from build123d import *

# Parameters (mm, degrees)
CROQUIS1_R              = 6
CROQUIS1_R_2            = 3
SALIENTE_EXTRUIR1_DEPTH = 2.5
CROQUIS3_W              = 4
CROQUIS3_H              = 4
CROQUIS3_R              = 0.75
SALIENTE_EXTRUIR2_DEPTH = 2.5
CORTAR_EXTRUIR1_DEPTH   = 5
MATRIZC1_COUNT          = 3


with BuildPart() as part:
    # Croquis1 → Saliente-Extruir1 (new, symmetric)
    with BuildSketch(Plane.XY):
        Circle(CROQUIS1_R)
        Circle(CROQUIS1_R_2, mode=Mode.SUBTRACT)
    extrude(amount=SALIENTE_EXTRUIR1_DEPTH, both=True)

    # Croquis3 → Saliente-Extruir2 (add, symmetric)
    with BuildSketch(Plane(origin=(0, 0, 0), x_dir=(0, 0, -1), z_dir=(1, 0, 0))):
        with Locations((0, 7)):
            Rectangle(CROQUIS3_W, CROQUIS3_H)
        with Locations((0, 7.5)):
            Circle(CROQUIS3_R, mode=Mode.SUBTRACT)
    saliente_extruir2 = extrude(amount=SALIENTE_EXTRUIR2_DEPTH, both=True)

    # Croquis4 → Cortar-Extruir1 (cut)
    with BuildSketch(Plane.XY.offset(2)):
        with BuildLine():
            Line((-1.25, 9), (1.25, 9))
            Line((1.25, 9), (1.25, 7.5))
            ThreePointArc((1.25, 7.5), (0.957106781, 6.792893219), (0.25, 6.5))
            Line((0.25, 6.5), (-0.25, 6.5))
            ThreePointArc((-0.25, 6.5), (-0.957106781, 6.792893219), (-1.25, 7.5))
            Line((-1.25, 7.5), (-1.25, 9))
        make_face()
    cortar_extruir1 = extrude(amount=-CORTAR_EXTRUIR1_DEPTH, mode=Mode.SUBTRACT)

    # MatrizC1: Saliente-Extruir2, Cortar-Extruir1 ×3 about axis
    matrizc1_axis = Axis((0, 0, 0), (0, 0, 1))
    add([saliente_extruir2.rotate(matrizc1_axis, i * 360 / MATRIZC1_COUNT) for i in range(1, MATRIZC1_COUNT)])
    add([cortar_extruir1.rotate(matrizc1_axis, i * 360 / MATRIZC1_COUNT) for i in range(1, MATRIZC1_COUNT)], mode=Mode.SUBTRACT)


solid = part.part
Verification items for the finished model (mm, model axes). A direction names the side the tool comes from. Coordinates: 2 decimals unless noted, no trailing zeros. Order: outer loops, then holes, each group sorted by start corner. A loop starts at its lowest first (then second) coordinate and runs counter-clockwise, first axis right, second up.
1. Sectioned sample at B-B, the plane y = 0. Record the cut outline in (x, z).
Results found:
outline: (-6, -2.5) - (-3, -2.5) - (-3, 2.5) - (-6, 2.5) - close; (3, -2.5) - (6, -2.5) - (6, 2.5) - (3, 2.5) - close
2. Set-up check for faces 1 (the face through (-6.655, -5.286, 0.028)), 2 (the face through (1.25, 8.4, 0)), 3 (the face through (6.673, -5.296, 0.028)): record each of +Z, -Z, +X, -X, +Y, -Y from which the full face is reachable in a straight line by a thin tool's end or side.
Results found:
face 1: +Z, -Z, -X
face 2: +Z, -Z, +Y
face 3: +Z, -Z, +X
3. Sectioned sample at D-D, the plane y = 2.75. Record the cut outline in (x, z).
Results found:
outline: (-5.33, -2.5) - (-1.2, -2.5) - (-1.2, 2.5) - (-5.33, 2.5) - close; (1.2, -2.5) - (5.33, -2.5) - (5.33, 2.5) - (1.2, 2.5) - close
4. Scan lines: line 1 (Z direction, x = 1.95, y = 7.5); line 2 (X direction, y = -5.5, z = -1.5); line 3 (X direction, y = 7, z = -0.75). Record each from-to range of solid material in increasing order.
Results found:
line 1: z = -2 to -0.75, 0.75 to 2
line 2: x = -7.03 to -4.53, -2.4 to 2.4, 4.53 to 7.03
line 3: x = -2.5 to -1.12, 1.12 to 2.5
5. Go/stop test with flat-tipped pins: pin 1 Ø1.7 at (x, y) = (6.5, -4.5) entering from -Z; pin 2 Ø2 at (y, z) = (7.5, 0) entering from +X; pin 3 Ø1.2 at (y, z) = (8, 0.5) entering from -X. Record where each tip stops, or that it passes through.
Results found:
pin 1: stops at z = -2
pin 2: stops at x = 2.5
pin 3: stops at x = -2.5
6. Release check for a two-part mould opening along Z. For faces 4 (the face through (5, -4, 2)), 5 (the face through (6.852, -6.131, 0.028)), 6 (the face through (-4.914, -5.024, 0.163)) record: +Z half, -Z half, draft (parallel to the pull), parting line (faces both ways), or undercut.
Results found:
face 4: +Z half
face 5: draft
face 6: undercut
7. Sectioned sample at A-A, the plane x = 0. Record the cut outline in (y, z), and give its area (3 significant figures).
Results found:
outline: (-6, -2.5) - (-3, -2.5) - (-3, 2.5) - (-6, 2.5) - close; (3, -2.5) - (6, -2.5) - (6, -2) - (6.5, -2) - (6.5, 2) - (6, 2) - (6, 2.5) - (3, 2.5) - close
area: 32.0 mm2
